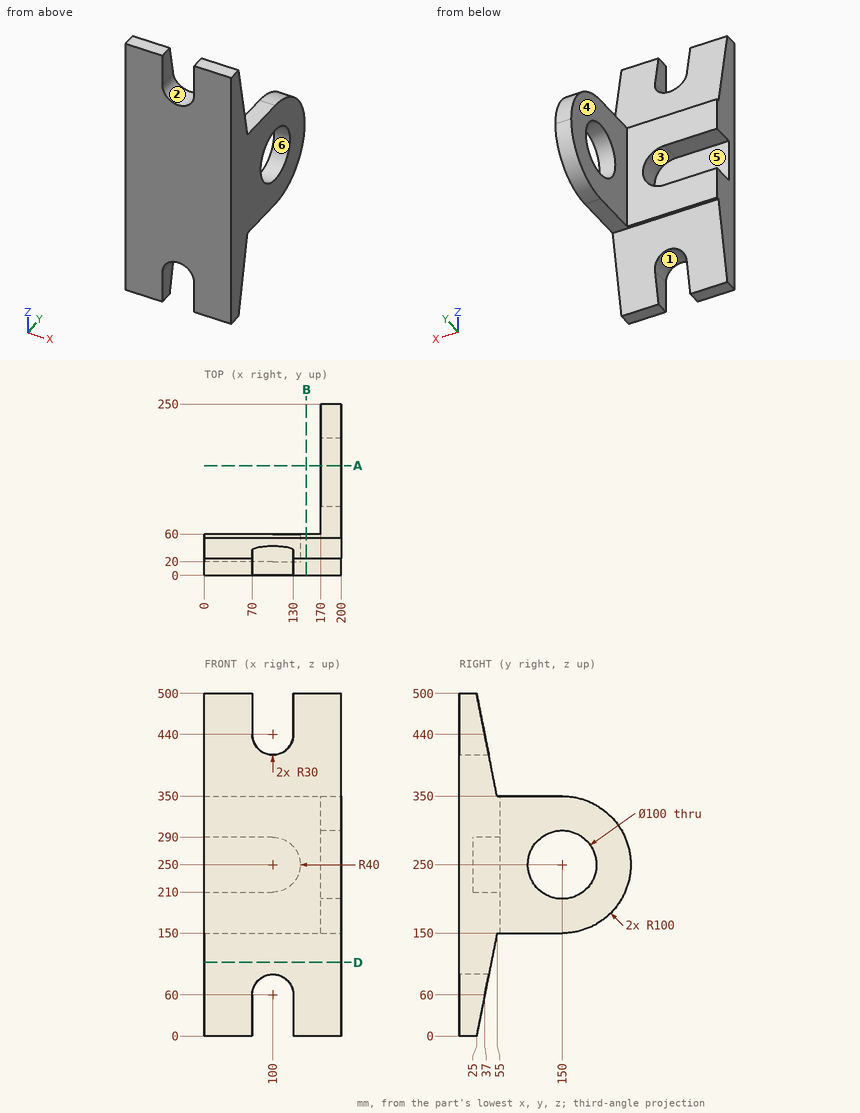
The figure shows three views and two pictorial views of one solid part (mm, origin at its lowest corner). Answer the questions. A direction names the side the tool comes from. Give positions to 0.01 mm unless a question says otherwise; leave off trailing zeros. Loops run counter-clockwise (first coordinate to the right, second up) from the corner with the lowest first, then second, coordinate; pieces in that order, holes last. Notation, with made-up numbers: (-22.75, 63.5) - (27.25, 63.5) arc R19 ccw to (27.25, 85.5) - close; hole circle Ø10 at (60, -22.75). An arc over 180 degrees is marked (long way). Answer in a Markdown table with one row per item.
(1) A tool of negligible diameter and unlimited length cuts with its end or side. For the marked faces 4, 5 and 6, from which of +Z, -Z, +X, -X, +Y, -Y can it reach the whole face along a straight path? Write none if from no direction.
Results list:
| item | result |
|---|---|
| face 4 | +Z, -Z, -X, +Y |
| face 5 | -X, +Y |
| face 6 | +X, -X |
(2) Flat-ended cylindrical pins translate along their axes: pin 1 Ø4 at (x, y) = (171.5, 214.5) entering from -Z; pin 2 Ø12 at (y, z) = (69, 201.5) entering from -X; pin 3 Ø3 at (x, z) = (103.5, 106) entering from +Y. Find the tip coordinate at first contact, or state that the pin passes through.
Results list:
| item | result |
|---|---|
| pin 1 | stops at z = 171.94 |
| pin 2 | stops at x = 170 |
| pin 3 | stops at y = 46.5 |
(3) For a pull along Z with two mould halves and no side action, classify the marked faces 1, 2 and 3 as pulls with the +Z half, pulls with the -Z half, needs draft (parallel to the pull), parting line crosses it, or undercut.
Results list:
| item | result |
|---|---|
| face 1 | pulls with the -Z half |
| face 2 | pulls with the +Z half |
| face 3 | undercut |
(4) Section D-D (z = 107.5) is taken. Give the vertices of the cut face in (x, y), and give its area (3 significant figures).
Results list:
| item | result |
|---|---|
| outline | (0, 0) - (200, 0) - (200, 46.5) - (0, 46.5) - close |
| area | 9,300 mm² |
(5) Section A-A (y = 160) is taken. Give the vertices of the cut face in (x, z), and give its area (3 significant figures).
Results list:
| item | result |
|---|---|
| outline | (170, 150.5) - (200, 150.5) - (200, 201.01) - (170, 201.01) - close; (170, 298.99) - (200, 298.99) - (200, 349.5) - (170, 349.5) - close |
| area | 3,030 mm² |
(6) Consider L1, parallel to Y at x = 184, z = 250; L2, parallel to Z at x = 98, y = 37; L3, parallel to Y at x = 56, z = 318.5. Determine where each line is inside the solid, lowest interval first. Write a range as [from, to].
Results list:
| item | result |
|---|---|
| L1 | y = [0, 100], [200, 250] |
| L2 | z = [89.93, 210], [290, 410.07] |
| L3 | y = [0, 60] |
(7) Section B-B (x = 149) is taken. Give the vertices of the cut face in (y, z), and give its area (3 significant figures).
Results list:
| item | result |
|---|---|
| outline | (0, 0) - (25, 0) - (55, 150) - (60, 150) - (60, 350) - (55, 350) - (25, 500) - (0, 500) - close |
| area | 24,000 mm² |
